Part model, mm, in its own coordinate system. Face numbers are marked on the shaded views. A direction names the side the tool comes from. Give positions to 0.01 mm unless a question says otherwise; leave off trailing zeros. Write each loop counter-clockwise with the first axis right and the second up, starting at its lowest first coordinate (ties: lowest second). Pieces come first, ordered by that corner, then holes.
Autodesk Inventor part; units mm, degrees
ref_plane "Start plane" through (0, 0, 0) normal (0, 0, 1) x (1, 0, 0)
ref_plane "End plane" through (0, 0, 12) normal (0, 0, 1) x (1, 0, 0)
ref_plane "YZ Plane" through (0, 0, 0) normal (1, 0, 0) x (0, 1, 0)
ref_plane "Start plane" through (0, 0, 0) normal (0, 0, 1) x (1, 0, 0)
ref_plane "End plane" through (0, 0, 12) normal (0, 0, 1) x (1, 0, 0)
sketch "Sketch2" plane through (0, 0, 0) normal (0, 0, 1) x (1, 0, 0)
  line L0 (-8.3, 28.5) -> (-11.5, 28.5)
  line L1 (-8.3, -5.1) -> (-8.3, 28.5)
  line L2 (28.5, -8.3) -> (-5.1, -8.3)
  line L3 (28.5, -11.5) -> (28.5, -8.3)
  line L4 (-5.1, -11.5) -> (28.5, -11.5)
  line L5 (-11.5, 28.5) -> (-11.5, -5.1)
  arc A0 (-8.3, -5.1) -> (-5.1, -8.3) centre (-5.1, -5.1) ccw
  arc A1 (-11.5, -5.1) -> (-5.1, -11.5) centre (-5.1, -5.1) ccw
  line L6 (0, 72.2651) -> (0, -13.5906) construction
  line L7 (-13.5906, 0) -> (72.2651, 0) construction
  point P0 (-8.3, -8.3)
  point P1 (-11.5, -11.5)
  dimension "d1" = 3.2
  dimension "d3" = 3.2
  dimension "d5" = 40
  dimension "d7" = 40
  dimension "d12" = 3.2
  dimension "d13" = 6.4
  dimension "d16" = 11.5
  dimension "d17" = 11.5
extrude "Body" add sketch "Sketch2" along normal up to surface (12 mm away) from surface at 0
sketch "Sketch3" plane through (0, 0, 0) normal (0, 0, 1) x (1, 0, 0)
  line L0 (0, 0) -> (10, 0)
ref_plane "Work Plane4" through (0, 0, 0) normal (0, -1, 0) x (1, 0, 0)
sketch "Sketch4" plane through (0, 0, 0) normal (0, -1, 0) x (1, 0, 0)
  line L0 (-2, 0) -> (12, 0)
  line L1 (-2, 12) -> (12, 12)
  dimension "d21" = 12
sketch "Sketch5" plane through (-8.3, -5.1, 12) normal (1, 0, 0) x (0, 0, -1)
  circle A0 centre (6, 10.6) radius 2
  line L0 (12, 33.6) -> (0, 33.6)
  line L1 (6, 33.6) -> (6, -25.4884) construction
  circle A1 centre (6, 25.6) radius 2
  line L2 (12, 0) -> (0, 0)
  line L3 (0, 0) -> (22.22, 0) construction
  point P0 (12, 5.1)
  dimension "d22" = 4
  dimension "d25" = 15
  dimension "d30" = 8
extrude "Extrusion2" cut sketch "Sketch5" against normal through all
sketch "Sketch6" plane through (28.5, -8.3, 12) normal (0, 1, 0) x (1, 0, 0)
  circle A0 centre (-5, 6) radius 2
  line L0 (0, 12) -> (0, 0)
  line L1 (0, 6) -> (-67.1079, 6) construction
  circle A1 centre (-10, 6) radius 2
  line L2 (-5, 4) -> (-10, 4)
  line L3 (-10, 4) -> (-10, 8)
  line L4 (-10, 8) -> (-5, 8)
  line L5 (-5, 8) -> (-5, 4)
  line L6 (0, 12) -> (0, 0)
  line L7 (0, 0) -> (-33.6, 0)
  line L8 (-33.6, 0) -> (-33.6, 12)
  line L9 (-39.1426, 12) -> (-33.6, 12)
  line L10 (-39.1426, 0) -> (-39.1426, 12)
  line L11 (-33.6, 0) -> (-39.1426, 0)
  line L12 (-33.6, 12) -> (0, 12)
  circle A2 centre (-20, 6) radius 2
  circle A3 centre (-25, 6) radius 2
  line L13 (-20, 4) -> (-25, 4)
  line L14 (-25, 4) -> (-25, 8)
  line L15 (-25, 8) -> (-20, 8)
  line L16 (-20, 8) -> (-20, 4)
  point P0 (-28.5, 12)
  dimension "d33" = 4
  dimension "d36" = 5
  dimension "d43" = 15
  dimension "d48" = 5
extrude "Extrusion3" cut sketch "Sketch6" against normal through all contours A0 L5 | L5 A0 | A0 L2 A1 L4 | L3 A1 | A1 L3 | A2 L16 | L16 A2 | A2 L13 A3 L15 | L14 A3 | A3 L14
equation "\"d1\" = ParT"
equation "\"d3\" = ParT"
equation "\"d12\" = ParT"
equation "\"d13\" = 2 * ParT"
equation "\"d16\" = ex"
equation "\"d17\" = ey"
equation "\"d8\" = G_L"
equation "\"ParT\" = 3.2"
equation "\"b\" = 40"
equation "\"ParH\" = 40"
equation "\"G_L\" = d21"
equation "\"ex\" = 11.5"
equation "\"ey\" = 11.5"
equation "\"G_OFFSET_START\" = 0"
equation "\"G_OFFSET_END\" = 0"
equation "\"d19\" = G_OFFSET_END + B_L"
equation "\"B_L\" = 12"
properties part number "JIS G 3350C - 3075     40x40-12" material "Steel, Mild"
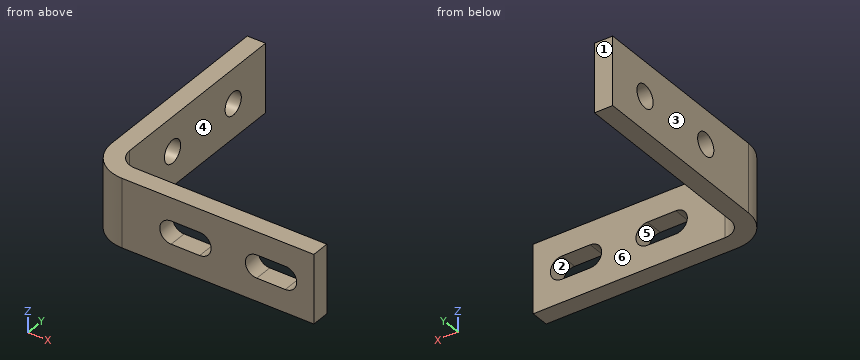
1) Saw through at A-A (z = 6). Write the cut outline in (x, y).
Check result:
outline: (-11.5, -5.1) arc R6.4 ccw to (-5.1, -11.5) - (1.5, -11.5) - (1.5, -8.3) - (-5.1, -8.3) arc R3.2 cw to (-8.3, -5.1) - (-8.3, 3.5) - (-11.5, 3.5) - close; (-11.5, 7.5) - (-8.3, 7.5) - (-8.3, 18.5) - (-11.5, 18.5) - close; (-11.5, 22.5) - (-8.3, 22.5) - (-8.3, 28.5) - (-11.5, 28.5) - close; (10.5, -11.5) - (16.5, -11.5) - (16.5, -8.3) - (10.5, -8.3) - close; (25.5, -11.5) - (28.5, -11.5) - (28.5, -8.3) - (25.5, -8.3) - close
2) 3-axis set-ups, long thin cutter, end or side, ignore diameter. For the marked faces 1 and 2: which of +Z, -Z, +X, -X, +Y, -Y reach the whole face in a straight line?
Check result:
face 1: +Z, -Z, +X, -X, +Y
face 2: +Y, -Y
3) Mould opens along X. For the marked faces 3, 4, 5 and 6 say: +X half, -X half, draft (parallel to the pull), parting line (faces both ways), or undercut.
Check result:
face 3: -X half
face 4: +X half
face 5: undercut
face 6: draft
4) Saw through at B-B (x = 7). Write the cut outline in (y, z).
Check result:
outline: (-11.5, 0) - (-8.3, 0) - (-8.3, 4) - (-11.5, 4) - close; (-11.5, 8) - (-8.3, 8) - (-8.3, 12) - (-11.5, 12) - close
5) Flat gauge pins, fed straight in: P1, Ø2, axis at x = 1, z = 10.5, coming from the +Y side; P2, Ø2, axis at y = 17, z = 10, coming from the +X side. Where does each tip first touch, or does it go through?
Check result:
P1: stops at y = -8.3
P2: stops at x = -8.3
6) Saw through at C-C (y = 21). Write the cut outline in (x, z).
Check result:
outline: (-11.5, 0) - (-8.3, 0) - (-8.3, 4.06) - (-11.5, 4.06) - close; (-11.5, 7.94) - (-8.3, 7.94) - (-8.3, 12) - (-11.5, 12) - close
7) Saw through at D-D (z = 2.5). Write the cut outline in (x, y).
Check result:
outline: (-11.5, -5.1) arc R6.4 ccw to (-5.1, -11.5) - (28.5, -11.5) - (28.5, -8.3) - (-5.1, -8.3) arc R3.2 cw to (-8.3, -5.1) - (-8.3, 28.5) - (-11.5, 28.5) - close
8) Drill centre lines: L1, parallel to Y at x = -1.5, z = 8; L2, parallel to Y at x = -10.25, z = 6; L3, parallel to Y at x = -9.8, z = 6. Where is each one in solid material? Low to high.
Check result:
L1: y = -11.5 to -8.3
L2: y = -8.9 to 3.5, 7.5 to 18.5, 22.5 to 28.5
L3: y = -9.44 to 3.5, 7.5 to 18.5, 22.5 to 28.5
